from build123d import *

# Parameters (mm, degrees)
BOSS_EXTRUDE1_DEPTH = 4.2
BOSS_EXTRUDE2_DEPTH = 5.8
CUT_EXTRUDE1_REACH  = 107.801
SKETCH2_R           = 3.375
LPATTERN1_COUNT     = 4
LPATTERN1_PITCH     = 20
CUT_EXTRUDE2_REACH  = 107.801
CUT_EXTRUDE3_DEPTH  = 15


with BuildPart() as part:
    # Sketch1 → Boss-Extrude1 (new body)
    with BuildSketch(Plane.XY):
        Polygon((40.2, 31.320919527), (25.2, 31.320919527), (25.2, -45), (40.2, -60), align=None)
        Polygon((62.2, 31.320919527), (40.2, 31.320919527), (40.2, -60), (40.2, -85), (62.2, -85), align=None)
    extrude(amount=BOSS_EXTRUDE1_DEPTH)

    # Sketch1<3> → Boss-Extrude2 (add)
    with BuildSketch(Plane.XY):
        Polygon((62.2, 31.320919527), (40.2, 31.320919527), (40.2, -60), (40.2, -85), (62.2, -85), align=None)
    extrude(amount=-BOSS_EXTRUDE2_DEPTH)

    # Sketch2 → Cut-Extrude1 (cut, up to next)
    with BuildSketch(Plane.XY.offset(4.2), mode=Mode.PRIVATE) as cut_extrude1_sk1:
        with Locations((51.2, 16.320919527)):
            Circle(SKETCH2_R)
    cut_extrude1_tool1 = extrude(cut_extrude1_sk1.sketch, amount=-CUT_EXTRUDE1_REACH, mode=Mode.PRIVATE) & part.part
    cut_extrude1 = cut_extrude1_tool1.solids().sort_by_distance((51.2, 16.32092, 4.2))[0]
    add(cut_extrude1, mode=Mode.SUBTRACT)

    # LPattern1: Cut-Extrude1 ×4
    with Locations(*[(0, -i * LPATTERN1_PITCH, 0) for i in range(1, LPATTERN1_COUNT)]):
        add(cut_extrude1, mode=Mode.SUBTRACT)

    # Sketch4 → Cut-Extrude2 (cut, up to next)
    with BuildSketch(Plane.XY.offset(4.2), mode=Mode.PRIVATE) as cut_extrude2_sk1:
        Polygon((52.2, -85), (40.2, -73), (40.2, -85), align=None)
    cut_extrude2_tool1 = extrude(cut_extrude2_sk1.sketch, amount=-CUT_EXTRUDE2_REACH, mode=Mode.PRIVATE) & part.part
    add(cut_extrude2_tool1.solids().sort_by_distance((44.2, -81, 4.2))[0], mode=Mode.SUBTRACT)

    # Sketch6 → Cut-Extrude3 (cut)
    with BuildSketch(Plane.ZY.offset(-25.2)):
        Polygon((3.7, -60), (0, -45), (0, -60), align=None)
    extrude(amount=-CUT_EXTRUDE3_DEPTH, mode=Mode.SUBTRACT)


solid = part.part
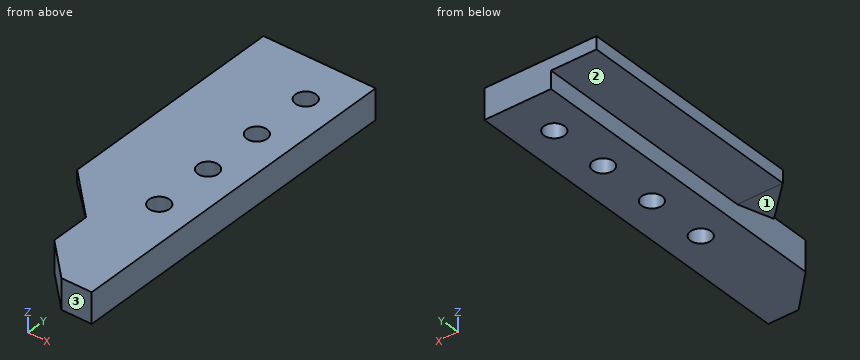
The listing builds one solid part. Answer for the finished solid, in the listing's coordinates (mm). Face numbers are marked on the shaded views. A direction names the side the tool comes from. Give positions to 0.01 mm unless a question says otherwise; leave off trailing zeros. Order: outer loops, then holes, each group sorted by start corner. A loop starts at its lowest first (then second) coordinate and runs counter-clockwise, first axis right, second up. Notation, with made-up numbers: (57.25, 20.5) - (70.25, 20.5) arc R19 ccw to (70.25, 37.5) - close; hole circle Ø8 at (26, 32.25). An arc over 180 degrees is marked (long way). Use one line per item in the form item = value.
1) Find section C-C on z = 1.25. Determine the outline of the cut face in (x, y) (3 decimals), and give its area (3 significant figures).
Verdict:
outline = (25.2, -45) - (30.268, -50.068) - (40.2, -50.068) - (40.2, -73) - (52.2, -85) - (62.2, -85) - (62.2, 31.321) - (25.2, 31.321) - close; hole circle Ø6.75 at (51.2, -43.679); hole circle Ø6.75 at (51.2, -23.679); hole circle Ø6.75 at (51.2, -3.679); hole circle Ø6.75 at (51.2, 16.321)
area = 3,550 mm^2
2) Find section A-A on x = 51.2. Determine the outline of the cut face in (y, z).
Verdict:
outline = (-84, -5.8) - (-47.05, -5.8) - (-47.05, 4.2) - (-84, 4.2) - close; (-40.3, -5.8) - (-27.05, -5.8) - (-27.05, 4.2) - (-40.3, 4.2) - close; (-20.3, -5.8) - (-7.05, -5.8) - (-7.05, 4.2) - (-20.3, 4.2) - close; (-0.3, -5.8) - (12.95, -5.8) - (12.95, 4.2) - (-0.3, 4.2) - close; (19.7, -5.8) - (31.32, -5.8) - (31.32, 4.2) - (19.7, 4.2) - close
3) Find section B-B on y = -5. Determine the outline of the cut face in (x, z).
Verdict:
outline = (25.2, 0) - (40.2, 0) - (40.2, -5.8) - (48.09, -5.8) - (48.09, 4.2) - (25.2, 4.2) - close; (54.31, -5.8) - (62.2, -5.8) - (62.2, 4.2) - (54.31, 4.2) - close
4) Consider probe 1 along Y at (x, z) = (51.2, 0.25); probe 2 along Y at (x, z) = (50.5, -1); probe 3 along X at (y, z) = (-24, -2.5). Determine where each line is inside the solid, lowest interval first. Write a range as [from, to].
Verdict:
probe_1 = [-84, -47.05], [-40.3, -27.05], [-20.3, -7.05], [-0.3, 12.95], [19.7, 31.32]
probe_2 = [-83.3, -46.98], [-40.38, -26.98], [-20.38, -6.98], [-0.38, 13.02], [19.62, 31.32]
probe_3 = [40.2, 47.84], [54.56, 62.2]
5) Each of these flat-tipped pins is pushed along its axis until it touches: pin 1 (5 mm diameter, centred on y = -16, z = -4, fed in from -X); pin 2 (12 mm diameter, centred on x = 31, y = 8.5, fed in from -Z). Where does it stop, or does it pass through?
Verdict:
pin_1 = 40.2
pin_2 = 0
6) For the marked faces 1, 2 and 3, determine the directions among +Z, -Z, +X, -X, +Y, -Y from which every point of the face is accessible in a straight line to the end or side of a thin tool.
Verdict:
face_1 = -Z, -X, -Y
face_2 = -Z, -X, +Y, -Y
face_3 = +Z, -Z, +X, -X, -Y
7) Find section D-D on x = 35. Determine the outline of the cut face in (y, z).
Verdict:
outline = (-54.8, 2.42) - (-45, 0) - (31.32, 0) - (31.32, 4.2) - (-54.8, 4.2) - close
